Design review of the part built by this model. Coordinates are the model's own, in mm. Face numbers are marked on the shaded views. A direction names the side the tool comes from. Coordinates: 2 decimals unless noted, no trailing zeros. Loops run counter-clockwise (first coordinate to the right, second up) from the corner with the lowest first, then second, coordinate; pieces in that order, holes last. Notation, with made-up numbers: M -25.5,86 L 28.5,86 A27 ccw 28.5,122 Z; hole C -3,89.25 d2. An arc over 180 degrees is marked long. Answer as a JSON object with one key per item and string values. Group by question number.
1. Insertion check: pin 1 (2 mm diameter, centred on x = -1.5, z = 2, fed in from +Y); pin 2 (0.9 mm diameter, centred on x = -13, y = 0, fed in from -Z); pin 3 (3 mm diameter, centred on x = -5.5, y = -1.5, fed in from +Z). Each pin has a flat end and moves straight along its axis. Give the tip position at first contact, or say it passes through.
2. Consider section A-A (x = -3.25). State the section outline as (y, z) points, then the cut area to 3 significant figures.
3. Machinability: for the marked faces 1 and 2, which of the approach directions +Z, -Z, +X, -X, +Y, -Y give a long, thin tool a straight path to every point of the face, cutting with its end or side? Answer none if there is none.
4. To check wall thickness, follow probe 1 along X at (y, z) = (-0.65, 0.2); probe 2 along Y at (x, z) = (-9, -0.9); probe 3 along X at (y, z) = (-1.3, -2.45). State the ranges of each line that lie inside material, in increasing order.
5. Consider section C-C (z = -2.05). State the section outline as (x, y) points.
6. Consider section B-B (y = 1.7). State the section outline as (x, z) points.
7. Draft analysis for pull direction Z (two halves, no side actions). For the marked faces 3, 4 and 5, state which applies: +Z half, -Z half, draft (parallel to the pull), parting line (faces both ways), or undercut.
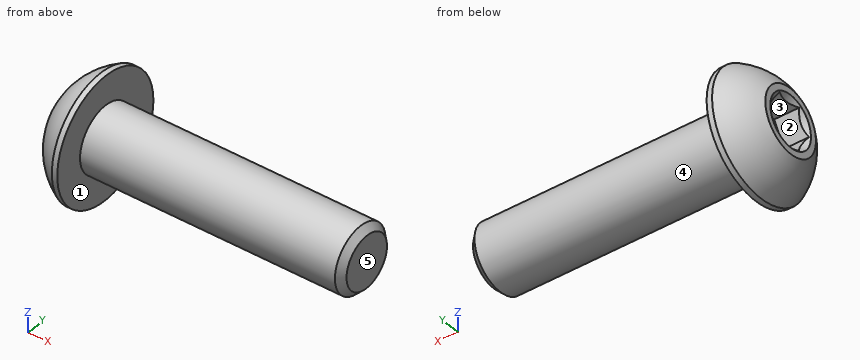
from build123d import *

# Parameters (mm, degrees)
SKETCH2_R           = 1.5
BOSS_EXTRUDE1_DEPTH = 12
CHAMFER1_SIZE       = 0.3
CUT_EXTRUDE1_DEPTH  = 1.2
SKETCH8_R           = 1.204700538
CUT_EXTRUDE2_DEPTH  = 1
CUT_EXTRUDE2_TAPER  = 45


with BuildPart() as part:
    # Sketch2 → Boss-Extrude1 (new body)
    with BuildSketch(Plane(origin=(0, 0, 0), x_dir=(0, 0, -1), z_dir=(1, 0, 0))):
        Circle(SKETCH2_R)
    extrude(amount=-BOSS_EXTRUDE1_DEPTH)

    # Chamfer1
    chamfer1_edges = [part.edges().sort_by_distance(p)[0] for p in [
        (0, 0, 1.5),
    ]]
    chamfer(chamfer1_edges, length=CHAMFER1_SIZE)

    # Sketch6 → Revolve1 (revolve)
    with BuildSketch(Plane.XY):
        with BuildLine():
            Line((-13.65, 0), (-13.65, 1.5))
            ThreePointArc((-13.65, 1.5), (-13.055944823, 2.284868705), (-12.25, 2.85))
            Line((-12.25, 2.85), (-12, 2.85))
            Line((-12, 2.85), (-12, 0))
            Line((-12, 0), (-13.65, 0))
        make_face()
    revolve(axis=Axis((-12, 0, 0), (-1, 0, 0)))

    # Sketch7 → Cut-Extrude1 (cut)
    with BuildSketch(Plane.ZY.offset(13.65)):
        Polygon((0, 1.154700538), (-1, 0.577350269), (-1, -0.577350269), (0, -1.154700538), (1, -0.577350269), (1, 0.577350269), align=None)
    extrude(amount=-CUT_EXTRUDE1_DEPTH, mode=Mode.SUBTRACT)

    # Sketch8 → Cut-Extrude2 (cut)
    with BuildSketch(Plane.ZY.offset(13.65)):
        Circle(SKETCH8_R)
    extrude(amount=-CUT_EXTRUDE2_DEPTH, taper=CUT_EXTRUDE2_TAPER, mode=Mode.SUBTRACT)


solid = part.part
Findings below:
{
 "1": {"pin 1": "stops at y = 1.12", "pin 2": "stops at z = -2.68", "pin 3": "stops at z = 1.5"},
 "2": {"outline": "C 0,0 d3", "area": "7.07 mm^2"},
 "3": {"face 1": "+X", "face 2": "-X"},
 "4": {"probe 1": "x = -12.45 to 0", "probe 2": "y = -1.2 to 1.2", "probe 3": "x = -12.4 to -12"},
 "5": {"outline": "M -12.25,-1.98 L -12,-1.98 L -12,1.98 L -12.25,1.98 A2.42 ccw Z"},
 "6": {"outline": "M -12.25,-2.29 L -12,-2.29 L -12,2.29 L -12.25,2.29 A2.68 ccw Z"},
 "7": {"face 3": "undercut", "face 4": "parting line", "face 5": "draft"}
}
